Verification items for the finished model (mm, model axes). A direction names the side the tool comes from. Give positions to 0.01 mm unless a question says otherwise; leave off trailing zeros. Loops run counter-clockwise (first coordinate to the right, second up) from the corner with the lowest first, then second, coordinate; pieces in that order, holes last. Notation, with made-up numbers: M 63,55 L 82,55 A28 cw 82,88 Z; hole C 85,55 d8. An arc over 180 degrees is marked long. Use a Markdown table: item, result.
from build123d import *

# Parameters (mm, degrees)
F1_DEPTH  = 41.9608
F2_R      = 1.9685
F3_DEPTH  = 14.606
F4_R      = 0.9525
F5_DEPTH  = 15.368
F6_R      = 3.048
F7_DEPTH  = 1.143
F8_R      = 1.524
F9_DEPTH  = 15.368
F10_R     = 4.0005
F11_DEPTH = 1.27


with BuildPart() as f1:
    # F0 (on Front) → F1 (new body)
    with BuildSketch(Plane.XZ):
        Polygon((0, -12.192), (0, 0), (11.43, 0), (11.43, 3.175), (-3.175, 3.175), (-3.175, -12.192), align=None)
    extrude(amount=F1_DEPTH)

    # F2 (on face) → F3 (cut, through all)
    with BuildSketch(Plane(origin=(-3.175, 0, 0), x_dir=(0, -1, 0), z_dir=(-1, 0, 0))):
        with Locations((5.5372, -3.302)):
            Circle(F2_R)
        with Locations((36.83, -3.683)):
            Circle(F2_R)
    extrude(amount=-F3_DEPTH, mode=Mode.SUBTRACT)

    # F4 (on face) → F5 (cut, through all)
    with BuildSketch(Plane.XY.offset(3.175)):
        with Locations((6.2738, -14.859)):
            Circle(F4_R)
    extrude(amount=-F5_DEPTH, mode=Mode.SUBTRACT)

    # F6 (on face) → F7 (cut)
    with BuildSketch(Plane(origin=(0, 0, 0), x_dir=(1, 0, 0), z_dir=(0, 0, -1))):
        with Locations((6.2738, 14.859)):
            Circle(F6_R)
    extrude(amount=-F7_DEPTH, mode=Mode.SUBTRACT)

    # F8 (on face) → F9 (cut, through all)
    with BuildSketch(Plane.XY.offset(3.175)):
        with Locations((5.969, -33.0708)):
            Circle(F8_R)
    extrude(amount=-F9_DEPTH, mode=Mode.SUBTRACT)

    # F10 (on face) → F11 (cut)
    with BuildSketch(Plane.XY.offset(3.175)):
        with Locations((5.969, -33.0708)):
            Circle(F10_R)
    extrude(amount=-F11_DEPTH, mode=Mode.SUBTRACT)


solid = f1.part
(1) Cross-section at A-A on y = -24. Record the cut outline in (x, z) (3 decimals).
Results below:
| item | result |
|---|---|
| outline | M -3.175,-12.192 L 0,-12.192 L 0,0 L 11.43,0 L 11.43,3.175 L -3.175,3.175 Z |
(2) Draft check along Y on faces 1 (the cylindrical face through (6.15, -13.915, 2.173)), 2 (the flat face through (-1, -41.961, -1)), 3 (the flat face through (11.43, -21, 2)). Enter one of: +Y half, -Y half, draft (parallel to the pull), parting line (faces both ways), or undercut.
Results below:
| item | result |
|---|---|
| face 1 | undercut |
| face 2 | -Y half |
| face 3 | draft |
(3) Material ranges on line 1 (Y direction, x = -0.5, z = -4); line 2 (Z direction, x = 10.25, y = -16) (3 decimals); line 3 (X direction, y = -30, z = -8.75) (3 decimals), recorded low to high.
Results below:
| item | result |
|---|---|
| line 1 | -41.96 to -38.77, -34.89 to -7.38, -3.7 to 0 |
| line 2 | 0 to 3.175 |
| line 3 | -3.175 to 0 |
(4) Set-up check for faces 4 (the flat face through (7, -16, 1.143)), 5 (the flat face through (0, -21, -6)), 6 (the flat face through (6, -35, 1.905)), 7 (the flat face through (-2, -21, -12.192)): record each of +Z, -Z, +X, -X, +Y, -Y from which the full face is reachable in a straight line by a thin tool's end or side.
Results below:
| item | result |
|---|---|
| face 4 | -Z |
| face 5 | -Z, +X, +Y, -Y |
| face 6 | +Z |
| face 7 | -Z, +X, -X, +Y, -Y |
(5) Cross-section at B-B on y = -4.5. Record the cut outline in (x, z) (3 decimals).
Results below:
| item | result |
|---|---|
| outline | M -3.175,-12.192 L 0,-12.192 L 0,-4.975 L -3.175,-4.975 Z; M -3.175,-1.629 L 0,-1.629 L 0,0 L 11.43,0 L 11.43,3.175 L -3.175,3.175 Z |
(6) Cross-section at D-D on x = 5.75. Record the cut outline in (y, z) (3 decimals), then the cut area to 3 significant figures.
Results below:
| item | result |
|---|---|
| outline | M -41.961,0 L -34.579,0 L -34.579,1.905 L -37.065,1.905 L -37.065,3.175 L -41.961,3.175 Z; M -31.563,0 L -17.862,0 L -17.862,1.143 L -15.655,1.143 L -15.655,3.175 L -29.076,3.175 L -29.076,1.905 L -31.563,1.905 Z; M -14.063,1.143 L -11.856,1.143 L -11.856,0 L 0,0 L 0,3.175 L -14.063,3.175 Z |
| area | 107 mm^2 |
(7) Gauge pin test, flat ends, axial feed: P1, Ø8, axis at x = 8, z = -7.5, coming from the +Y side; P2, Ø4, axis at x = 5.97, y = -33.07, coming from the -Z side; P3, Ø6.5, axis at x = 5.97, y = -33.07, coming from the +Z side (3 decimals); P4, Ø5, axis at y = -15, z = -6, coming from the +X side. Record the tip position at first contact, or that the pin passes through.
Results below:
| item | result |
|---|---|
| P1 | through |
| P2 | z = 0 |
| P3 | z = 1.905 |
| P4 | x = 0 |
(8) Cross-section at C-C on x = 8. Record the cut outline in (y, z) (3 decimals), then the cut area to 3 significant figures.
Results below:
| item | result |
|---|---|
| outline | M -41.961,0 L -17.371,0 L -17.371,1.143 L -12.347,1.143 L -12.347,0 L 0,0 L 0,3.175 L -29.624,3.175 L -29.624,1.905 L -36.517,1.905 L -36.517,3.175 L -41.961,3.175 Z |
| area | 119 mm^2 |
